```python
from build123d import *

# Parameters (mm, degrees)
F0_W     = 930
F0_H     = 400
F1_DEPTH = 18
F2_SIZE  = 17.99999


# Not quite as in the source:
# - a fillet or chamfer is up to 0.001 mm smaller than in the source, because OpenCascade refuses the exact size


with BuildPart() as f1:
    # F0 (on Top) → F1 (new body)
    with BuildSketch(Plane.XY):
        Rectangle(F0_W, F0_H)
    extrude(amount=-F1_DEPTH)

    # F2 (size 18 in the source; OpenCascade refuses exactly that, so slightly less here)
    f2_edges = [f1.edges().sort_by_distance(p)[0] for p in [
        (0, -200, -18),
    ]]
    chamfer(f2_edges, length=F2_SIZE)


solid = f1.part
```
Here's how the part is built. I have some questions about the finished solid (model axes, mm). Coordinates: 2 decimals unless noted, no trailing zeros. Order: outer loops, then holes, each group sorted by start corner. A loop starts at its lowest first (then second) coordinate and runs counter-clockwise, first axis right, second up. Notation, with made-up numbers: M 35,88 L 41,88 A27 cw 41,120 Z; hole C 12.5,41.25 d1. An arc over 180 degrees is marked long. Answer as a JSON object with one key per item and string values. Group by question number.
(1) For pin 1 (10 mm diameter, centred on x = 362.5, z = -7.5, fed in from -Y), with a flat end and sliding along its axis, tell me the tip position at first contact or that it passes through.
(2) If we mould it in two halves opening along Z, with no side actions, what happens to faces 1 (the face through (-7, 3, 0)), 2 (the face through (-7, 12, -18)), 3 (the face through (465, -3, -9))? For each: released by +Z, released by -Z, zero draft, split by the parting line, or undercut.
(3) Suppose I cut it at B-B, the plane z = -15.25. Please give me the cut outline in (x, y), then the cut area to 3 significant figures.
(4) I need wall thicknesses on probe 1 along Y at (x, z) = (85, -5); probe 2 along Y at (x, z) = (-248, -3.5). Which ranges of each line are inside material? Lowest first, please.
Values found:
{
 "1": {"pin 1": "stops at y = -197.5"},
 "2": {"face 1": "released by +Z", "face 2": "released by -Z", "face 3": "zero draft"},
 "3": {"outline": "M -465,-184.75 L 465,-184.75 L 465,200 L -465,200 Z", "area": "358,000 mm^2"},
 "4": {"probe 1": "y = -195 to 200", "probe 2": "y = -196.5 to 200"}
}
